from build123d import *

# Parameters (mm, degrees)
PAD003_DEPTH    = 6.5
SKETCH016_R     = 10.5
POCKET005_DEPTH = 37.001
POCKET006_DEPTH = 20.001
SKETCH018_R     = 3.4
POCKET007_DEPTH = 20
PAD001_DEPTH    = 21.5
PAD002_DEPTH    = 6
PAD_DEPTH       = 26
SKETCH010_R     = 3.4
POCKET_DEPTH    = 20
POCKET001_DEPTH = 26.001
POCKET002_DEPTH = 41.501
POCKET003_DEPTH = 40.001
POCKET004_DEPTH = 7


with BuildPart() as body006:
    # Sketch015 → Pad003 (new body)
    with BuildSketch(Plane.XZ.offset(-19)):
        with BuildLine():
            Line((7.845523, 28.25), (9, 26))
            Line((9, 26), (9, 0))
            Line((9, 0), (20, 0))
            Line((20, 0), (20, 26))
            Line((16.75, 26), (20, 26))
            ThreePointArc((11, 31.75), (12.684136, 27.684136), (16.75, 26))
            Line((11, 31.75), (11, 37))
            Line((11, 37), (7, 37))
            Line((7, 37), (7, 31.75))
            ThreePointArc((7, 31.75), (7.214378, 29.949659), (7.845523, 28.25))
        make_face()
    extrude(amount=-PAD003_DEPTH)

    # Sketch016 → Pocket005 (cut, through all)
    with BuildSketch(Plane.XY):
        with Locations((20, 10.5)):
            Circle(SKETCH016_R)
    extrude(amount=POCKET005_DEPTH, mode=Mode.SUBTRACT)

    # Sketch017 → Pocket006 (cut, through all)
    with BuildSketch(Plane.YZ):
        Polygon((20.5, 0), (20.5, 26), (19, 30), (19, 0), align=None)
        Polygon((25.5, 26), (24.5, 30), (24.5, 37), (25.5, 37), align=None)
    extrude(amount=POCKET006_DEPTH, mode=Mode.SUBTRACT)

    # Sketch018 → Pocket007 (cut)
    with BuildSketch(Plane.XZ.offset(-41.5)):
        with Locations((7, 8)):
            Circle(SKETCH018_R)
        with BuildLine():
            ThreePointArc((35.404163, 5.595837), (33, 11.4), (30.595837, 5.595837))
            Line((30.595837, 5.595837), (33, 3.191674))
            Line((33, 3.191674), (35.404163, 5.595837))
        make_face()
    extrude(amount=POCKET007_DEPTH, mode=Mode.SUBTRACT)


with BuildPart() as obj1:
    # Sketch006 → Pad001 (new body)
    with BuildSketch(Plane.XZ):
        with BuildLine():
            ThreePointArc((7, 11.4), (3.85881, 9.301124), (4.595837, 5.595837))
            Line((10.191674, 0), (4.595837, 5.595837))
            Line((10.191674, 0), (29.808326, 0))
            Line((29.808326, 0), (35.404163, 5.595837))
            ThreePointArc((35.404163, 5.595837), (36.14119, 9.301124), (33, 11.4))
            Line((33, 11.4), (7, 11.4))
        make_face()
    extrude(amount=-PAD001_DEPTH)


with BuildPart() as sideboltboss:
    # Sketch007 → Pad002 (new body)
    with BuildSketch(Plane.XY):
        with BuildLine():
            Line((5, 0), (5, 10.5))
            ThreePointArc((20, 25.5), (9.393398, 21.106602), (5, 10.5))
            ThreePointArc((20, 25.5), (24.242641, 27.257359), (26, 31.5))
            Line((26, 41.5), (26, 31.5))
            Line((40, 41.5), (26, 41.5))
            Line((40, 22.571068), (40, 41.5))
            ThreePointArc((40, 22.571068), (36.299458, 17.032815), (35, 10.5))
            Line((35, 0), (35, 10.5))
            Line((5, 0), (35, 0))
        make_face()
    extrude(amount=PAD002_DEPTH)


with BuildPart() as fusion001:
    # Sketch → Pad (new body)
    with BuildSketch(Plane.XY):
        with BuildLine():
            ThreePointArc((35, 10.5), (20, 25.5), (5, 10.5))
            Line((5, 0), (5, 10.5))
            Line((5, 0), (35, 0))
            Line((35, 0), (35, 10.5))
        make_face()
    extrude(amount=PAD_DEPTH)

    # Fusion: union obj1, SideBoltBoss
    add(obj1.part)
    add(sideboltboss.part)

    # Sketch010 → Pocket (cut)
    with BuildSketch(Plane.XZ.offset(-41.5)):
        with Locations((7, 8)):
            Circle(SKETCH010_R)
        with BuildLine():
            ThreePointArc((35.404163, 5.595837), (33, 11.4), (30.595837, 5.595837))
            Line((30.595837, 5.595837), (33, 3.191674))
            Line((33, 3.191674), (35.404163, 5.595837))
        make_face()
    extrude(amount=POCKET_DEPTH, mode=Mode.SUBTRACT)

    # Sketch011 → Pocket001 (cut, through all)
    with BuildSketch(Plane.XY):
        with BuildLine():
            ThreePointArc((28, 3.699265), (20, 21), (12, 3.699265))
            Line((12, 3.699265), (12, 0))
            Line((12, 0), (28, 0))
            Line((28, 3.699265), (28, 0))
        make_face()
    extrude(amount=POCKET001_DEPTH, mode=Mode.SUBTRACT)

    # Sketch012 → Pocket002 (cut, through all)
    with BuildSketch(Plane.XZ.offset(-41.5)):
        with BuildLine():
            ThreePointArc((5.833274, 9.166726), (7, 6.35), (8.166726, 9.166726))
            Line((7.5, 9.833452), (8.166726, 9.166726))
            Line((6.5, 9.833452), (7.5, 9.833452))
            Line((5.833274, 9.166726), (6.5, 9.833452))
        make_face()
        with BuildLine():
            ThreePointArc((31.833274, 9.166726), (33, 6.35), (34.166726, 9.166726))
            Line((33.5, 9.833452), (34.166726, 9.166726))
            Line((32.5, 9.833452), (33.5, 9.833452))
            Line((31.833274, 9.166726), (32.5, 9.833452))
        make_face()
    extrude(amount=POCKET002_DEPTH, mode=Mode.SUBTRACT)

    # Sketch013 → Pocket003 (cut, through all)
    with BuildSketch(Plane.YZ):
        Polygon((0, 16), (10.5, 16), (20.5, 26), (0, 26), align=None)
        with BuildLine():
            ThreePointArc((37.333274, 4.166726), (38.5, 1.35), (39.666726, 4.166726))
            Line((39, 4.833452), (39.666726, 4.166726))
            Line((38, 4.833452), (39, 4.833452))
            Line((37.333274, 4.166726), (38, 4.833452))
        make_face()
        with BuildLine():
            ThreePointArc((41.5, 3), (40.62132, 5.12132), (38.5, 6))
            Line((35.5, 6), (38.5, 6))
            Line((35.5, 9), (35.5, 6))
            Line((44.5, 9), (35.5, 9))
            Line((44.5, 0), (44.5, 9))
            Line((41.5, 0), (44.5, 0))
            Line((41.5, 3), (41.5, 0))
        make_face()
    extrude(amount=POCKET003_DEPTH, mode=Mode.SUBTRACT)

    # Sketch014 → Pocket004 (cut)
    with BuildSketch(Plane.YZ.offset(40)):
        Polygon((38.5, 8), (43.5, 8), (43.5, 3), (38.5, 3), (36.85, 3), (36.85, 8), align=None)
    extrude(amount=-POCKET004_DEPTH, mode=Mode.SUBTRACT)

    # Fusion001: union Body006
    add(body006.part)


solid = fusion001.part
Here's how the part is built. I have some questions about the finished solid (model axes, mm). A direction names the side the tool comes from. Coordinates: 2 decimals unless noted, no trailing zeros. Loops run counter-clockwise (first coordinate to the right, second up) from the corner with the lowest first, then second, coordinate; pieces in that order, holes last.
1. Imagine slicing it at B-B, the plane y = 7.5. Please give me the cut outline in (x, z), and give its area (3 significant figures).
2. Imagine slicing it at D-D, the plane z = 21. Please give me the cut outline in (x, y), and give its area (3 significant figures).
3. For faces 1 (the flat face through (8.415, 22.537, 27.141)), 2 (the flat face through (34.19, 29.28, 4.38)), 3 (the flat face through (8, 5, 16)), which set-ups out of +Z, -Z, +X, -X, +Y, -Y let a thin tool reach every point of the face, with its end or its side?
4. If we mould it in two halves opening along Z, with no side actions, what happens to faces 4 (the cylindrical face through (32.95, 10.9, 6.35)), 5 (the cylindrical face through (28.67, 40.64, 5.1)), 6 (the cylindrical face through (3.637, 10.599, 8.499)), 7 (the flat face through (37, 36.85, 4))? For each: pulls with the +Z half, pulls with the -Z half, needs draft (parallel to the pull), parting line crosses it, or undercut.
5. Imagine slicing it at C-C, the plane y = 34. Please give me the cut outline in (x, z).
6. Imagine slicing it at A-A, the plane z = 8. Please give me the cut outline in (x, y).
7. I need wall thicknesses on L1, parallel to X at y = 19.5, z = 7; L2, parallel to X at y = 10.5, z = 9; L3, parallel to X at y = 10.5, z = 12. Which ranges of each line are inside material? Lowest first, please.
8. For P1, Ø5, axis at x = 15, z = 23, coming from the +Y side; P2, Ø0.8, axis at x = 32.5, y = 20, coming from the +Z side; P3, Ø7.5, axis at x = 9, y = 7, coming from the +Z side; P4, Ø1.5, axis at x = 9, y = 8.5, coming from the -Z side, each with a flat end and sliding along its axis, tell me the tip position at first contact or that it passes through.
Taken from the geometry:
1. outline: (4.6, 5.6) - (5, 5.19) - (5, 0) - (9.94, 0) - (9.94, 16) - (5, 16) - (5, 10.75) arc R3.4 ccw to start; (30.06, 0) - (35, 0) - (35, 5.19) - (35.4, 5.6) arc R3.4 ccw to (35, 10.75) - (35, 16) - (30.06, 16) - close; hole (5.83, 9.17) arc R1.65 ccw (long way) to (8.17, 9.17) - (7.5, 9.83) - (6.5, 9.83) - close; hole (31.83, 9.17) arc R1.65 ccw (long way) to (34.17, 9.17) - (33.5, 9.83) - (32.5, 9.83) - close
1. area: 151 mm2
2. outline: (5.86, 15.5) - (10.77, 15.5) arc R10.5 cw to (29.23, 15.5) - (34.14, 15.5) arc R15 ccw to (20, 25.5) - (9, 25.5) - (9, 20.7) arc R15 ccw to start
2. area: 150 mm2
3. face 1: -X, +Y, -Y
3. face 2: +Z, +Y
3. face 3: +Z, +X, -X, -Y
4. face 4: undercut
4. face 5: pulls with the +Z half
4. face 6: parting line crosses it
4. face 7: needs draft
5. outline: (26, 0) - (40, 0) - (40, 6) - (35.75, 6) arc R3.4 cw to (35.4, 5.6) - (33, 3.19) - (30.6, 5.6) arc R3.4 cw to (30.25, 6) - (26, 6) - close
6. outline: (3.6, 0) - (5.35, 0) - (5.35, 21.5) - (3.6, 21.5) - close; (8.65, 0) - (12, 0) - (12, 3.7) arc R10.5 cw (long way) to (28, 3.7) - (28, 0) - (31.35, 0) - (31.35, 21.5) - (29.6, 21.5) - (29.6, 22.03) arc R15 ccw to (20, 25.5) - (10.4, 25.5) - (10.4, 21.5) - (8.65, 21.5) - close; (34.65, 0) - (36.4, 0) - (36.4, 21.5) - (34.65, 21.5) - close
7. L1: x = 3.75 to 5.69, 8.31 to 14.59, 25.41 to 31.69, 34.31 to 36.25
7. L2: x = 3.75 to 5.69, 8.31 to 9.5, 30.5 to 31.69, 34.31 to 36.25
7. L3: x = 5 to 9.5, 30.5 to 35
8. P1: stops at y = 25.5
8. P2: stops at z = 11.4
8. P3: stops at z = 16.25
8. P4: stops at z = 0
